```python
from build123d import *

# Parameters (mm, degrees)
SKETCH1_R           = 42
SKETCH1_R_2         = 34
SKETCH1_R_3         = 1.75
BOSS_EXTRUDE1_DEPTH = 10
SKETCH2_R           = 2.55
CUT_EXTRUDE1_DEPTH  = 7


with BuildPart() as part:
    # Sketch1 → Boss-Extrude1 (new body)
    with BuildSketch(Plane.XY):
        Circle(SKETCH1_R)
        Circle(SKETCH1_R_2, mode=Mode.SUBTRACT)
        with Locations((0, 38)):
            Circle(SKETCH1_R_3, mode=Mode.SUBTRACT)
        with Locations((38, 0)):
            Circle(SKETCH1_R_3, mode=Mode.SUBTRACT)
        with Locations((0, -38)):
            Circle(SKETCH1_R_3, mode=Mode.SUBTRACT)
        with Locations((-38, 0)):
            Circle(SKETCH1_R_3, mode=Mode.SUBTRACT)
    extrude(amount=BOSS_EXTRUDE1_DEPTH)

    # Sketch2 → Cut-Extrude1 (cut)
    with BuildSketch(Plane.XY.offset(10)):
        with Locations((0, 38)):
            Circle(SKETCH2_R)
        with Locations((38, 0)):
            Circle(SKETCH2_R)
        with Locations((0, -38)):
            Circle(SKETCH2_R)
        with Locations((-38, 0)):
            Circle(SKETCH2_R)
    extrude(amount=-CUT_EXTRUDE1_DEPTH, mode=Mode.SUBTRACT)


solid = part.part
```
Could you check a few things on this model? Use its own coordinates, in mm. A direction names the side the tool comes from. Round coordinates to 2 decimals unless told otherwise and drop trailing zeros. Loops run counter-clockwise (first coordinate to the right, second up) from the corner with the lowest first, then second, coordinate; pieces in that order, holes last.
Q1. For P1, Ø4.5, axis at x = 0, y = -38, coming from the +Z side; P2, Ø3, axis at y = -11.5, z = 2, coming from the -X side; P3, Ø4, axis at y = -29.5, z = 3, coming from the +X side, each with a flat end and sliding along its axis, tell me the tip position at first contact or that it passes through.
Q2. On a 3-axis mill with a long thin cutter (end or side, diameter ignored), from which of +Z, -Z, +X, -X, +Y, -Y can I reach the whole of each face in a straight line? I mean faces 1 (the cylindrical face through (-0.38, -39.71, 1.48)), 2 (the cylindrical face through (35.452, 0.112, 6.549)). Say none if no direction works.
Q3. I want a section at C-C (z = 1.5). Write out the boundary of the cut face in (x, y).
Q4. I want a section at A-A (x = 0). Write out the boundary of the cut face in (y, z), and give its area (3 significant figures).
Q5. I want a section at D-D (x = 10). Write out the boundary of the cut face in (y, z), and give its area (3 significant figures).
Q6. Please list where these lines run through material, in increasing order: L1, parallel to Y at x = 0, z = 6.75; L2, parallel to Y at x = 38, z = 2; L3, parallel to X at y = -29, z = 6.5.
Q7. Thinking about a two-plate mould opening in X: for faces 3 (the flat face through (34.03, -2.92, 0)), 4 (the flat face through (-1, -40, 3)), 5 (the cylindrical face through (40.06, 12.62, 4.93)), which applies, pulls with the +X half, pulls with the -X half, needs draft (parallel to the pull), parting line crosses it, or undercut?
Answer below:
1. P1: stops at z = 3
1. P2: stops at x = -40.79
1. P3: stops at x = 31.75
2. face 1: +Z, -Z
2. face 2: +Z
3. outline: circle Ø84 at (0, 0); hole circle Ø3.5 at (-38, 0); hole circle Ø68 at (0, 0); hole circle Ø3.5 at (0, -38); hole circle Ø3.5 at (0, 38); hole circle Ø3.5 at (38, 0)
4. outline: (-42, 0) - (-39.75, 0) - (-39.75, 3) - (-40.55, 3) - (-40.55, 10) - (-42, 10) - close; (-36.25, 0) - (-34, 0) - (-34, 10) - (-35.45, 10) - (-35.45, 3) - (-36.25, 3) - close; (34, 0) - (36.25, 0) - (36.25, 3) - (35.45, 3) - (35.45, 10) - (34, 10) - close; (39.75, 0) - (42, 0) - (42, 10) - (40.55, 10) - (40.55, 3) - (39.75, 3) - close
4. area: 67.6 mm2
5. outline: (-40.79, 0) - (-32.5, 0) - (-32.5, 10) - (-40.79, 10) - close; (32.5, 0) - (40.79, 0) - (40.79, 10) - (32.5, 10) - close
5. area: 166 mm2
6. L1: y = -42 to -40.55, -35.45 to -34, 34 to 35.45, 40.55 to 42
6. L2: y = -17.89 to -1.75, 1.75 to 17.89
6. L3: x = -30.38 to -17.75, 17.75 to 30.38
7. face 3: needs draft
7. face 4: undercut
7. face 5: parting line crosses it
